Here's the drawing with two shaded views (mm, measured from the low corner). I have some questions. Round coordinates to 2 decimals unless told otherwise and drop trailing zeros. Loops run counter-clockwise (first coordinate to the right, second up) from the corner with the lowest first, then second, coordinate; pieces in that order, holes last. Notation, with made-up numbers: (0, 63) - (50, 63) arc R30 cw to (50, 101) - close; hole circle Ø10 at (35.25, 22.25). An arc over 180 degrees is marked (long way). Use one line per item in the form item = value.
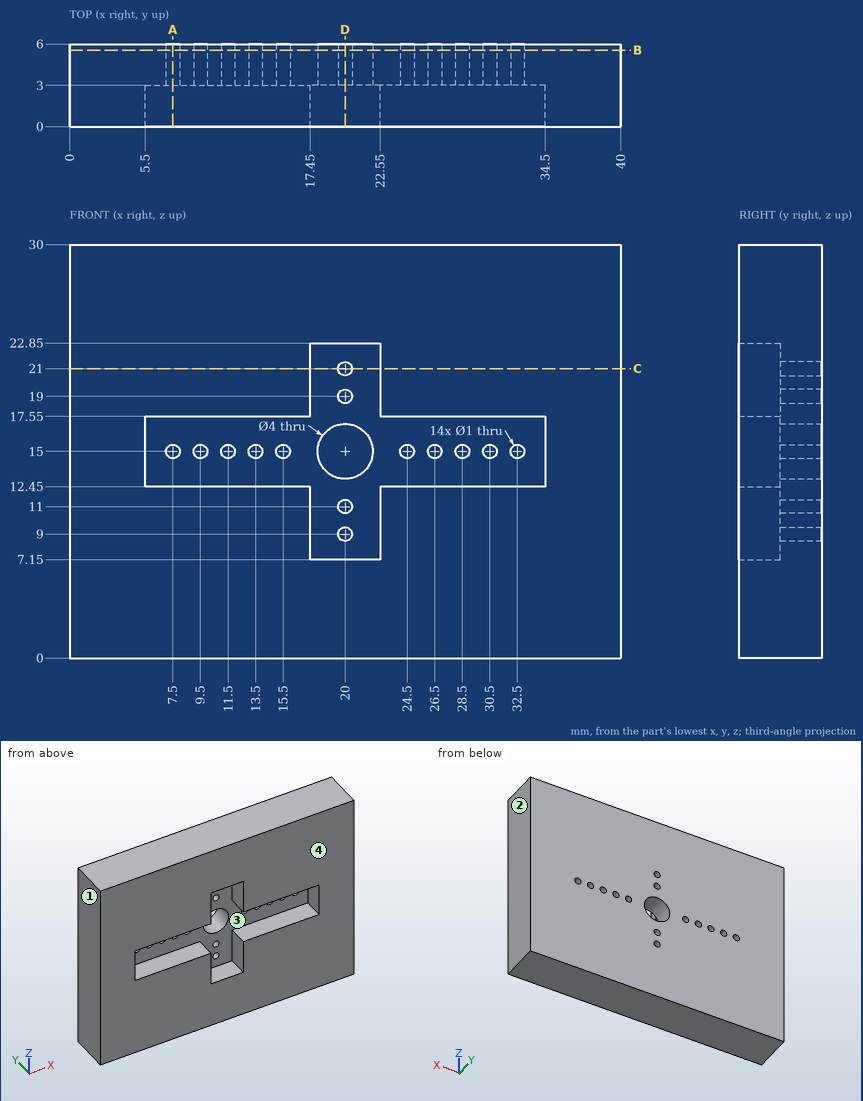
1. Please list where these lines run through material, in increasing order: line 1 along X through (y, z) = (0.75, 18.75); line 2 along X through (y, z) = (4.65, 11); line 3 along Z through (x, y) = (14.5, 2.1).
Solution:
line_1 = 0 to 17.45, 22.55 to 40
line_2 = 0 to 19.5, 20.5 to 40
line_3 = 0 to 12.45, 17.55 to 30
2. We'd pull the mould along X, two halves only. Please class the marked faces 1, 2, 3 and 4: +X half, -X half, draft (parallel to the pull), parting line (faces both ways), or undercut.
Solution:
face_1 = -X half
face_2 = +X half
face_3 = undercut
face_4 = draft
3. If we section it at A-A, the plane x = 7.5: Write out the boundary of the cut face in (y, z), plus the area to 3 significant figures.
Solution:
outline = (0, 0) - (6, 0) - (6, 14.5) - (3, 14.5) - (3, 12.45) - (0, 12.45) - close; (0, 17.55) - (3, 17.55) - (3, 15.5) - (6, 15.5) - (6, 30) - (0, 30) - close
area = 162 mm^2
4. If we section it at C-C, the plane z = 21: Write out the boundary of the cut face in (x, y).
Solution:
outline = (0, 0) - (17.45, 0) - (17.45, 3) - (19.5, 3) - (19.5, 6) - (0, 6) - close; (20.5, 3) - (22.55, 3) - (22.55, 0) - (40, 0) - (40, 6) - (20.5, 6) - close
5. If we section it at B-B, the plane y = 5.55: Count the separate pieces of the cut face and the enclosed holes in it, plus the area to 3 significant figures.
Solution:
separate_pieces = 1
enclosed_holes = 15
area = 1,180 mm^2
6. If we section it at D-D, the plane x = 20: Write out the boundary of the cut face in (y, z), plus the area to 3 significant figures.
Solution:
outline = (0, 0) - (6, 0) - (6, 8.5) - (3, 8.5) - (3, 7.15) - (0, 7.15) - close; (0, 22.85) - (3, 22.85) - (3, 21.5) - (6, 21.5) - (6, 30) - (0, 30) - close; (3, 9.5) - (6, 9.5) - (6, 10.5) - (3, 10.5) - close; (3, 11.5) - (6, 11.5) - (6, 13) - (3, 13) - close; (3, 17) - (6, 17) - (6, 18.5) - (3, 18.5) - close; (3, 19.5) - (6, 19.5) - (6, 20.5) - (3, 20.5) - close
area = 109 mm^2
